```python
from build123d import *

# Parameters (mm, degrees)
EXTRUDE_1_DEPTH     = 4.4
SKETCH_2_R          = 1.6
CUT_EXTRUDE_1_DEPTH = 10
EXTRUDE_2_DEPTH     = 4.4


with BuildPart() as part:
    # 草图1 → 凸台-拉伸1 (new body)
    with BuildSketch(Plane.XY):
        Polygon((5, 19.4), (5, 15), (-5, 15), (-5, 19.4), (-13, 19.4), (-13, 15), (-17.5, 15), (-17.5, -15), (-13, -15), (-13, -19.4), (-5, -19.4), (-5, -15), (5, -15), (5, -19.4), (13, -19.4), (13, -15), (17.5, -15), (17.5, 15), (13, 15), (13, 19.4), align=None)
    extrude(amount=EXTRUDE_1_DEPTH)

    # 草图2 → 切除-拉伸1 (cut)
    with BuildSketch(Plane.XY.offset(4.4)):
        Circle(SKETCH_2_R)
    extrude(amount=-CUT_EXTRUDE_1_DEPTH, mode=Mode.SUBTRACT)

    # 草图3 → 凸台-拉伸2 (add)
    with BuildSketch(Plane.XY.offset(4.4)):
        Polygon((10, 88.5), (10, 84.1), (13, 84.1), (13, 15), (-13, 15), (-13, 84.1), (-10, 84.1), (-10, 88.5), align=None)
    extrude(amount=-EXTRUDE_2_DEPTH)


solid = part.part
```
For this review, take the finished solid that the model builds, in its own axes (mm). A direction names the side the tool comes from. Coordinates: 2 decimals unless noted, no trailing zeros. Order: outer loops, then holes, each group sorted by start corner. A loop starts at its lowest first (then second) coordinate and runs counter-clockwise, first axis right, second up. Notation, with made-up numbers: (35, 50.5) -> (40, 50.5) arc R15 ccw to (40, 67.5) -> close; hole circle Ø3 at (48, 62). An arc over 180 degrees is marked (long way). Answer as CSV lines item,"result".
Q1. Clearance check with flat-ended pins moving along their axes: pin 1 Ø2 at (y, z) = (64.5, 2.5) entering from -X; pin 2 Ø2 at (x, z) = (16, 1) entering from +Y; pin 3 Ø2.5 at (x, z) = (-11, 3) entering from +Y; pin 4 Ø2 at (y, z) = (86.5, 2.5) entering from -X. State where each tip first meets the part, or that it passes through.
Model answer:
pin 1,"stops at x = -13"
pin 2,"stops at y = 15"
pin 3,"stops at y = 88.5"
pin 4,"stops at x = -10"
Q2. We need section A-A (x = 0). State the section outline as (y, z) points, plus the area to 3 significant figures.
Model answer:
outline,"(-15, 0) -> (-1.6, 0) -> (-1.6, 4.4) -> (-15, 4.4) -> close; (1.6, 0) -> (88.5, 0) -> (88.5, 4.4) -> (1.6, 4.4) -> close"
area,"441 mm2"
Q3. Wall thickness on line 1 along Y through (x, z) = (0, 2.9); line 2 along X through (y, z) = (43, 4.25); line 3 along Y through (x, z) = (-3, 3.5): over which ranges is each line inside the solid? List them lowest first. Write a range as [from, to].
Model answer:
line 1,"y = [-15, -1.6], [1.6, 88.5]"
line 2,"x = [-13, 13]"
line 3,"y = [-15, 88.5]"
Q4. We need section B-B (y = 0). State the section outline as (x, z) points, plus the area to 3 significant figures.
Model answer:
outline,"(-17.5, 0) -> (-1.6, 0) -> (-1.6, 4.4) -> (-17.5, 4.4) -> close; (1.6, 0) -> (17.5, 0) -> (17.5, 4.4) -> (1.6, 4.4) -> close"
area,"140 mm2"
Q5. For faces 1 (the face through (0, -15, 2)), 2 (the face through (15, 15, 2)), 3 (the face through (15, -15, 2)), list the 3-axis set-ups (+Z, -Z, +X, -X, +Y, -Y) from which the entire face can be reached by the end or side of a thin tool; tool diameter is ignored.
Model answer:
face 1,"+Z, -Z, -Y"
face 2,"+Z, -Z, +X, +Y"
face 3,"+Z, -Z, +X, -Y"
Q6. We need section C-C (z = 2.3). State the section outline as (x, y) points.
Model answer:
outline,"(-17.5, -15) -> (-13, -15) -> (-13, -19.4) -> (-5, -19.4) -> (-5, -15) -> (5, -15) -> (5, -19.4) -> (13, -19.4) -> (13, -15) -> (17.5, -15) -> (17.5, 15) -> (13, 15) -> (13, 84.1) -> (10, 84.1) -> (10, 88.5) -> (-10, 88.5) -> (-10, 84.1) -> (-13, 84.1) -> (-13, 15) -> (-17.5, 15) -> close; hole circle Ø3.2 at (0, 0)"
Q7. We need section D-D (y = 50). State the section outline as (x, z) points, plus the area to 3 significant figures.
Model answer:
outline,"(-13, 0) -> (13, 0) -> (13, 4.4) -> (-13, 4.4) -> close"
area,"114 mm2"
Q8. Draft analysis for pull direction X (two halves, no side actions). For faces 4 (the face through (-5, -17, 2)), 5 (the face through (11, 84.1, 2)), 6 (the face through (13, 50, 2)), 7 (the face through (-13, 49, 2)), state which applies: released by +X, released by -X, zero draft, split by the parting line, or undercut.
Model answer:
face 4,"undercut"
face 5,"zero draft"
face 6,"released by +X"
face 7,"released by -X"
